Source: CAD feature listing. Evaluate the final solid. Frame: model axes, mm. A direction names the side the tool comes from. Give positions to 0.01 mm unless a question says otherwise; leave off trailing zeros. Write each loop counter-clockwise with the first axis right and the second up, starting at its lowest first coordinate (ties: lowest second). Pieces come first, ordered by that corner, then holes. Notation, with made-up numbers: M -17,59 L 31,59 A29 ccw 31,86 Z; hole C 77,-8.5 d7. An arc over 180 degrees is marked long. Return JSON: item names as keys, results as strings.
```python
from build123d import *

# Parameters (mm, degrees)
SKETCH_2_R      = 2.5
SKETCH_2_R_2    = 2
EXTRUDE_1_DEPTH = 1
SKETCH_3_R      = 2.5
SKETCH_3_R_2    = 2
EXTRUDE_2_DEPTH = 1
SKETCH_5_R      = 2.5
SKETCH_5_R_2    = 2
EXTRUDE_3_DEPTH = 1


with BuildPart() as part:
    # Эскиз2 → Бобышка-Вытянуть1 (new body)
    with BuildSketch(Plane(origin=(0, 0, 0), x_dir=(1, 0, 0), z_dir=(0, 1, 0))):
        with BuildLine():
            Line((0, -45), (0, 0))
            Line((0, 0), (45, 0))
            ThreePointArc((45, 0), (31.819805153, -31.819805153), (0, -45))
        make_face()
        with Locations(Location((25, -25, 0), (0, 0, 270))):
            Circle(SKETCH_2_R, mode=Mode.SUBTRACT)
        with Locations(Location((14.393398282, -35.606601718, 0), (0, 0, 270))):
            Circle(SKETCH_2_R_2, mode=Mode.SUBTRACT)
        with Locations(Location((35.606601718, -14.393398282, 0), (0, 0, 90))):
            Circle(SKETCH_2_R_2, mode=Mode.SUBTRACT)
    extrude(amount=EXTRUDE_1_DEPTH)

    # Эскиз3 → Бобышка-Вытянуть2 (add)
    with BuildSketch(Plane.XY):
        with BuildLine():
            Line((0, 45), (0, 0))
            Line((0, 0), (45, 0))
            ThreePointArc((45, 0), (31.819805153, 31.819805153), (0, 45))
        make_face()
        with Locations((25, 25)):
            Circle(SKETCH_3_R, mode=Mode.SUBTRACT)
        with Locations((14.393398282, 35.606601718)):
            Circle(SKETCH_3_R_2, mode=Mode.SUBTRACT)
        with Locations(Location((35.606601718, 14.393398282, 0), (0, 0, 180))):
            Circle(SKETCH_3_R_2, mode=Mode.SUBTRACT)
    extrude(amount=EXTRUDE_2_DEPTH)

    # Эскиз5 → Бобышка-Вытянуть3 (add)
    with BuildSketch(Plane(origin=(0, 0, 0), x_dir=(0, 0, -1), z_dir=(1, 0, 0))):
        with BuildLine():
            Line((0, 45), (0, 0))
            Line((0, 0), (-45, 0))
            ThreePointArc((-45, 0), (-31.819805153, 31.819805153), (0, 45))
        make_face()
        with Locations((-25, 25)):
            Circle(SKETCH_5_R, mode=Mode.SUBTRACT)
        with Locations((-14.393398282, 35.606601718)):
            Circle(SKETCH_5_R_2, mode=Mode.SUBTRACT)
        with Locations(Location((-35.606601718, 14.393398282, 0), (0, 0, 180))):
            Circle(SKETCH_5_R_2, mode=Mode.SUBTRACT)
    extrude(amount=EXTRUDE_3_DEPTH)


solid = part.part
```
1) Draft query along X for faces 1 (the face through (27.48, 0.49, 24.67)), 2 (the face through (1, 18, 18)), 3 (the face through (18, 0, 17)), 4 (the face through (33.7, 13.79, 0.49)). Return one class per face: released by +X, released by -X, zero draft, split by the parting line, or undercut.
Numbers:
{"face 1": "undercut", "face 2": "released by +X", "face 3": "zero draft", "face 4": "undercut"}
2) Cut plane A-A, the plane y = 26.5. Return the cut outline in (x, z).
Numbers:
{"outline": "M 0,0 L 23,0 L 23,1 L 1,1 L 1,23 L 0,23 Z; M 0,27 L 1,27 L 1,36.37 L 0,36.37 Z; M 27,0 L 36.37,0 L 36.37,1 L 27,1 Z"}
3) Line query: line 1 (Z direction, x = 3.5, y = 36). Output: solid intervals per line, ascending. Write a range as [from, to].
Numbers:
{"line 1": "z = [0, 1]"}
4) Contact query for flat-ended pins moving along their axis: pin 1 Ø12 at (x, z) = (39, 24.5) entering from +Y; pin 2 Ø5 at (y, z) = (24, 16) entering from +X; pin 3 Ø10 at (x, y) = (22.5, 33) entering from +Z. Output: stop coordinate, or through.
Numbers:
{"pin 1": "stops at y = 1", "pin 2": "stops at x = 1", "pin 3": "stops at z = 1"}
5) Cut plane B-B, the plane z = 25. Return the cut outline in (x, y), then the cut area to 3 significant figures.
Numbers:
{"outline": "M 0,0 L 22.5,0 L 22.5,1 L 1,1 L 1,22.5 L 0,22.5 Z; M 0,27.5 L 1,27.5 L 1,37.42 L 0,37.42 Z; M 27.5,0 L 37.42,0 L 37.42,1 L 27.5,1 Z", "area": "63.8 mm²"}
6) Cut plane C-C, the plane x = 9. Return the cut outline in (y, z).
Numbers:
{"outline": "M 0,0 L 44.09,0 L 44.09,1 L 1,1 L 1,44.09 L 0,44.09 Z"}
7) Cut plane D-D, the plane z = 38.5. Return the cut outline in (x, y), then the cut area to 3 significant figures.
Numbers:
{"outline": "M 0,0 L 23.3,0 L 23.3,1 L 1,1 L 1,23.3 L 0,23.3 Z", "area": "45.6 mm²"}
8) Set-up query: faces 5 (the face through (15.316, 33.832, 0.493)), 6 (the face through (18, 18, 1)). Return all of +Z, -Z, +X, -X, +Y, -Y with unobstructed straight access to the full face (end or side cutting, diameter ignored); none if empty.
Numbers:
{"face 5": "+Z, -Z", "face 6": "+Z, +X, +Y"}
